The listing builds one solid part. Answer for the finished solid, in the listing's coordinates (mm). Face numbers are marked on the shaded views. A direction names the side the tool comes from. Round coordinates to 2 decimals unless told otherwise and drop trailing zeros. Loops run counter-clockwise (first coordinate to the right, second up) from the corner with the lowest first, then second, coordinate; pieces in that order, holes last. Notation, with made-up numbers: (-13.5, -28.75) -> (40.5, -28.75) arc R23 cw to (40.5, 4.25) -> close; hole circle Ø10 at (88.25, -39.75). An arc over 180 degrees is marked (long way). Use a Markdown table: item, result. Add a question column.
Q1. Section A-A on x = -3 is taken. Give the vertices of the cut face in (y, z).
Q2. Which of the six approach directions +Z, -Z, +X, -X, +Y, -Y give full straight-line access (tool end or side, diameter ignored) to the marked faces 1, 2 and 3?
Q3. Section D-D on x = -5.5 is taken. Give the vertices of the cut face in (y, z), then the cut area to 3 significant figures.
Q4. For a pull along Z with two mould halves and no side action, classify the marked faces 4, 5 and 6 as released by +Z, released by -Z, zero draft, split by the parting line, or undercut.
Q5. Given pin 1 Ø1 at (x, y) = (-6, 0) entering from -Z; pin 2 Ø3 at (y, z) = (3, -3.5) entering from +X; pin 3 Ø3 at (y, z) = (0.5, -1.5) entering from -X; pin 4 Ø4 at (y, z) = (0.5, 4) entering from -X, each flat-ended and moving along its own axis, determine where each tip first touches the part or whether it passes through.
Q6. Section B-B on y = -1 is taken. Give the vertices of the cut face in (x, z).
Q7. Section C-C on z = 3.5 is taken. Give the vertices of the cut face in (x, y), then the cut area to 3 significant figures.
Q8. Consider line 1 (Z direction, x = 3, y = 7.25); line 2 (Y direction, x = 0, z = -3.75); line 3 (Y direction, x = 0, z = -1). Determine where each line is inside the solid, lowest interval first.
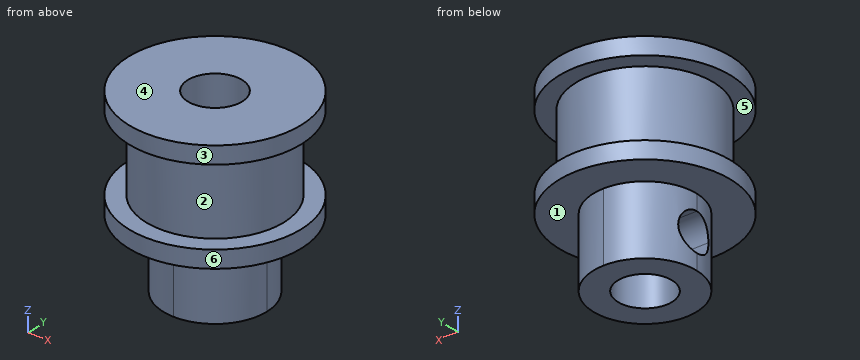
from build123d import *

# Parameters (mm, degrees)
F0_R         = 6.35
F1_DEPTH     = 7
F2_R         = 7.9375
F3_DEPTH     = 1.5875
F4_R         = 7.9375
F5_DEPTH     = 1.5875
F6_W         = 9.525
F6_H         = 9.525
F7_DEPTH     = 6.35
F8_R         = 2.5
F9_DEPTH     = 16.525
F11_REACH    = 16.5631366107
F12_T1_DEPTH = 18.25625


# Not quite as in the source:
# - a fillet or chamfer that OpenCascade refuses, or shapes differently, is made with other operations: its cross-section is extruded or revolved along the edge and cut away or added


with BuildPart() as f1:
    # F0 (on Top) → F1 (new body)
    with BuildSketch(Plane.XY):
        Circle(F0_R)
    extrude(amount=F1_DEPTH)

    # F2 (on face) → F3 (join)
    with BuildSketch(Plane.XY.offset(7)):
        Circle(F2_R)
    extrude(amount=F3_DEPTH)

    # F4 (on face) → F5 (join)
    with BuildSketch(Plane(origin=(0, 0, 0), x_dir=(1, 0, 0), z_dir=(0, 0, -1))):
        Circle(F4_R)
    extrude(amount=F5_DEPTH)

    # F6 (on face) → F7 (join)
    with BuildSketch(Plane(origin=(0, 0, -1.5875), x_dir=(1, 0, 0), z_dir=(0, 0, -1))):
        Rectangle(F6_W, F6_H)
    extrude(amount=F7_DEPTH)

    # F8 (on face) → F9 (cut, through all)
    with BuildSketch(Plane(origin=(0, 0, -7.9375), x_dir=(1, 0, 0), z_dir=(0, 0, -1))):
        Circle(F8_R)
    extrude(amount=-F9_DEPTH, mode=Mode.SUBTRACT)

    f11_end = f1.faces().sort_by_distance((-2.5, 0, 0.325))[0]
    # F10 (on face) → F11 (cut, up to a face of the model that its end follows)
    with BuildSketch(Plane(origin=(-4.7625, 0, 0), x_dir=(0, -1, 0), z_dir=(-1, 0, 0))):
        with BuildLine():
            ThreePointArc((0, -3.0353), (-1.7272, -4.7625), (0, -6.4897))
            Line((0, -6.4897), (0, -3.0353))
        make_face()
        with BuildLine():
            Line((0, -3.0353), (0, -6.4897))
            ThreePointArc((0, -6.4897), (1.2213148325, -5.9838148325), (1.7272, -4.7625))
            ThreePointArc((1.7272, -4.7625), (1.2213148325, -3.5411851675), (0, -3.0353))
        make_face()
    f11_long = extrude(amount=-F11_REACH, mode=Mode.PRIVATE)
    add(split(f11_long, bisect_by=f11_end, keep=Keep.ALL, mode=Mode.PRIVATE).solids().sort_by_distance((-4.7625, 0, -4.7625))[0], mode=Mode.SUBTRACT)

    # F12: fillet of radius 4.7625 on 4 edges, made by hand

    # F12_s2 → F12_t1 (cut)
    with BuildSketch(Plane.XY.offset(-19.84375)):
        with BuildLine():
            ThreePointArc((-4.7625, 0), (-3.3675960454, -3.3675960454), (0, -4.7625))
            Line((0, -4.7625), (-4.7625, -4.7625))
            Line((-4.7625, -4.7625), (-4.7625, 0))
        make_face()
        with BuildLine():
            ThreePointArc((-4.7625, 0), (-3.3675960454, 3.3675960454), (0, 4.7625))
            Line((0, 4.7625), (-4.7625, 4.7625))
            Line((-4.7625, 4.7625), (-4.7625, 0))
        make_face()
        with BuildLine():
            ThreePointArc((0, 4.7625), (3.3675960454, 3.3675960454), (4.7625, 0))
            Line((4.7625, 0), (4.7625, 4.7625))
            Line((4.7625, 4.7625), (0, 4.7625))
        make_face()
        with BuildLine():
            ThreePointArc((4.7625, 0), (3.3675960454, -3.3675960454), (0, -4.7625))
            Line((0, -4.7625), (4.7625, -4.7625))
            Line((4.7625, -4.7625), (4.7625, 0))
        make_face()
    extrude(amount=F12_T1_DEPTH, mode=Mode.SUBTRACT)


solid = f1.part
Checked values:
| question | item | result |
|---|---|---|
| 1 | outline | (-7.35, -1.59) -> (-3.7, -1.59) -> (-3.7, -7.94) -> (3.7, -7.94) -> (3.7, -1.59) -> (7.35, -1.59) -> (7.35, 0) -> (5.6, 0) -> (5.6, 7) -> (7.35, 7) -> (7.35, 8.59) -> (-7.35, 8.59) -> (-7.35, 7) -> (-5.6, 7) -> (-5.6, 0) -> (-7.35, 0) -> close; hole circle Ø3.45 at (0, -4.76) |
| 2 | face 1 | -Z |
| 2 | face 2 | none |
| 2 | face 3 | +Z, -Z |
| 3 | outline | (-5.72, -1.59) -> (5.72, -1.59) -> (5.72, 0) -> (3.17, 0) -> (3.17, 7) -> (5.72, 7) -> (5.72, 8.59) -> (-5.72, 8.59) -> (-5.72, 7) -> (-3.17, 7) -> (-3.17, 0) -> (-5.72, 0) -> close |
| 3 | area | 80.8 mm2 |
| 4 | face 4 | released by +Z |
| 4 | face 5 | undercut |
| 4 | face 6 | zero draft |
| 5 | pin 1 | stops at z = -1.59 |
| 5 | pin 2 | stops at x = 4.52 |
| 5 | pin 3 | stops at x = -7.94 |
| 5 | pin 4 | stops at x = -6.35 |
| 6 | outline | (-7.87, -1.59) -> (-4.66, -1.59) -> (-4.66, -3.35) -> (-2.29, -3.35) -> (-2.29, 8.59) -> (-7.87, 8.59) -> (-7.87, 7) -> (-6.27, 7) -> (-6.27, 0) -> (-7.87, 0) -> close; (-4.66, -7.94) -> (-2.29, -7.94) -> (-2.29, -6.17) -> (-4.66, -6.17) -> close; (2.29, -7.94) -> (4.66, -7.94) -> (4.66, -1.59) -> (7.87, -1.59) -> (7.87, 0) -> (6.27, 0) -> (6.27, 7) -> (7.87, 7) -> (7.87, 8.59) -> (2.29, 8.59) -> close |
| 7 | outline | circle Ø12.7 at (0, 0); hole circle Ø5 at (0, 0) |
| 7 | area | 107 mm2 |
| 8 | line 1 | z = -1.59 to 0, 7 to 8.59 |
| 8 | line 2 | y = -4.76 to -2.5, 2.5 to 4.76 |
| 8 | line 3 | y = -7.94 to -2.5, 2.5 to 7.94 |
